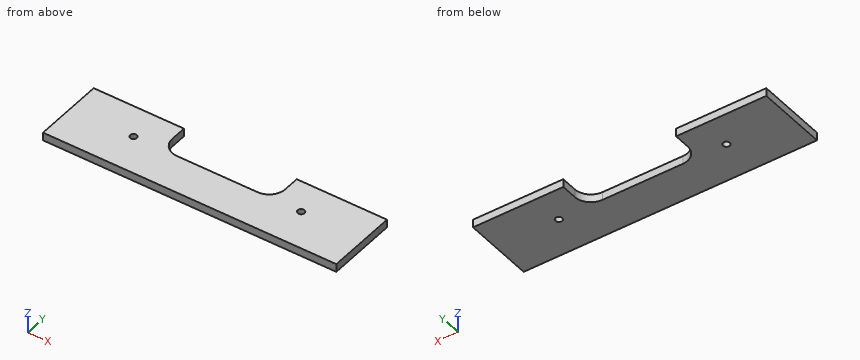
from build123d import *

# Parameters (mm, degrees)
SKIZZE1_W                       = 182
SKIZZE1_H                       = 50
AUFSATZ_LINEAR_AUSTRAGEN1_DEPTH = 5
M5_GEWINDEBOHRUNG1_D            = 4.2
M5_GEWINDEBOHRUNG1_DEPTH        = 14
M5_GEWINDEBOHRUNG1_TIP          = 1.2618073
SKIZZE4_W                       = 70
SKIZZE4_H                       = 20
SKIZZE4_W_2                     = 182
SKIZZE4_H_2                     = 6
SCHNITT_LINEAR_AUSTRAGEN1_DEPTH = 10
VERRUNDUNG2_R                   = 10


with BuildPart() as part:
    # Skizze1 → Aufsatz-Linear austragen1 (new body)
    with BuildSketch(Plane.XY):
        Rectangle(SKIZZE1_W, SKIZZE1_H)
    extrude(amount=AUFSATZ_LINEAR_AUSTRAGEN1_DEPTH)

    # M5 Gewindebohrung1
    with Locations(Plane.XY.offset(5)):
        with Locations((52, 5), (-52, 5)):
            Hole(M5_GEWINDEBOHRUNG1_D / 2, depth=M5_GEWINDEBOHRUNG1_DEPTH)
            with Locations((0, 0, -(M5_GEWINDEBOHRUNG1_DEPTH + M5_GEWINDEBOHRUNG1_TIP / 2))):  # 118° drill point
                Cone(0, M5_GEWINDEBOHRUNG1_D / 2, M5_GEWINDEBOHRUNG1_TIP, mode=Mode.SUBTRACT)

    # Skizze4 → Schnitt-Linear austragen1 (cut)
    with BuildSketch(Plane.XY.offset(5)):
        with Locations((0, 15)):
            Rectangle(SKIZZE4_W, SKIZZE4_H)
        with Locations((0, -22)):
            Rectangle(SKIZZE4_W_2, SKIZZE4_H_2)
    extrude(amount=-SCHNITT_LINEAR_AUSTRAGEN1_DEPTH, mode=Mode.SUBTRACT)

    # Verrundung2
    verrundung2_edges = [part.edges().sort_by_distance(p)[0] for p in [
        (-35, 5, 2.5),
        (35, 5, 2.5),
    ]]
    fillet(verrundung2_edges, radius=VERRUNDUNG2_R)


solid = part.part
Read the model definition and answer for the solid it produces. Units are mm, in the model's axes. Give positions to 0.01 mm unless a question says otherwise; leave off trailing zeros. Write each loop counter-clockwise with the first axis right and the second up, starting at its lowest first coordinate (ties: lowest second). Pieces come first, ordered by that corner, then holes. Notation, with made-up numbers: (19.25, -14) -> (77.25, -14) arc R25 ccw to (77.25, 12) -> close; hole circle Ø4 at (14.25, 7.5). An arc over 180 degrees is marked (long way). Answer as a JSON object with one key per item and string values. Group by question number.
1) Find section D-D (x = -1.5). Write down the section's boundary in (y, z).
2) Find section C-C (z = 3.6). Write down the section's boundary in (x, y).
3) Find section B-B (y = 20.5). Write down the section's boundary in (x, z), and give its area (3 significant figures).
4) This flat-tipped pin is pushed along its axis until it touches: P1, Ø1.5, axis at x = -4, z = 2, coming from the +Y side. Where does it stop, or does it pass through?
5) Find section A-A (x = 52). Write down the section's boundary in (y, z), and give its area (3 significant figures).
6) Consider L1, parallel to Y at x = 52, z = 1.15; L2, parallel to X at y = 4.5, z = 4.8; L3, parallel to Y at x = -11, z = 3.1. Determine where each line is inside the solid, lowest interval first. Write a range as from..to.
Values follow:
{
 "1": {"outline": "(-19, 0) -> (5, 0) -> (5, 5) -> (-19, 5) -> close"},
 "2": {"outline": "(-91, -19) -> (91, -19) -> (91, 25) -> (35, 25) -> (35, 15) arc R10 cw to (25, 5) -> (-25, 5) arc R10 cw to (-35, 15) -> (-35, 25) -> (-91, 25) -> close; hole circle Ø4.2 at (-52, 5); hole circle Ø4.2 at (52, 5)"},
 "3": {"outline": "(-91, 0) -> (-35, 0) -> (-35, 5) -> (-91, 5) -> close; (35, 0) -> (91, 0) -> (91, 5) -> (35, 5) -> close", "area": "560 mm2"},
 "4": {"P1": "stops at y = 5"},
 "5": {"outline": "(-19, 0) -> (2.9, 0) -> (2.9, 5) -> (-19, 5) -> close; (7.1, 0) -> (25, 0) -> (25, 5) -> (7.1, 5) -> close", "area": "199 mm2"},
 "6": {"L1": "y = -19..2.9, 7.1..25", "L2": "x = -91..-54.04, -49.96..49.96, 54.04..91", "L3": "y = -19..5"}
}
